Could you check a few things on this model? Use its own coordinates, in mm. A direction names the side the tool comes from. Give positions to 0.01 mm unless a question says otherwise; leave off trailing zeros. Loops run counter-clockwise (first coordinate to the right, second up) from the corner with the lowest first, then second, coordinate; pieces in that order, holes last. Notation, with made-up numbers: M 76,-19.75 L 92,-19.75 A14 ccw 92,-4.75 Z; hole C 62,8.5 d8. An arc over 180 degrees is marked long. Answer in a Markdown table with one row per item. Add a question column.
1. If we section it at A-A on y = 21.5: List the corners of the cut face in (x, z) for me (3 decimals).
2. Thinking about a two-plate mould opening in X: for faces 1 (the flat face through (-4.802, 20, 2)), 2 (the flat face through (25.698, 39, 2)), 3 (the flat face through (32.198, 20, 2)), 4 (the flat face through (13, -6.855, 2)), which applies, released by +X, released by -X, zero draft, split by the parting line, or undercut?
3. I need wall thicknesses on line 1 along Y through (x, z) = (11, 2.7); line 2 along X through (y, z) = (35.5, 0.5); line 3 along Y through (x, z) = (6, 2.4). Which ranges of each line are inside material? Lowest first, please. Write a range as from..to.
4. If we section it at B-B on x = 9.5: List the corners of the cut face in (y, z) for me (3 decimals), then the cut area to 3 significant figures.
5. If we section it at C-C on y = 39: List the corners of the cut face in (x, z) for me (3 decimals).
6. Which directions (+Z, -Z, +X, -X, +Y, -Y) give clear straight access to the entire face, cutting with the end or side of a thin tool? Please do faces 5 (the flat face through (8, 20.82, 2)), 6 (the flat face through (13, 47.32, 2)).
7. If we section it at D-D on x = 23.5: List the corners of the cut face in (y, z) for me (3 decimals).
8. I'm going to push a flat-ended pin straight in: pin 1 Ø1.2 at (x, y) = (-0.8, 11.57) entering from -Z. Where does the tip first touch, or does it pass through?
```python
from build123d import *

# Parameters (mm, degrees)
F0_W     = 37
F0_H     = 54.175
F0_W_2   = 6
F0_H_2   = 3.175
F0_R     = 1
F0_W_3   = 8.325
F0_H_3   = 23.5
F0_W_4   = 10
F0_H_4   = 10
F0_R_2   = 1.2
F1_DEPTH = 3.175


# Not quite as in the source:
# - a length typed as a fraction of an inch, garbled in the dataset ("3 / 203.2 mm" for 3/8 in), is restored
# - a feature names something its author has since deleted; it is built from what else it names


with BuildPart() as f1:
    # F0 (on Top) → F1 (new body)
    with BuildSketch(Plane.XY):
        with Locations((13.6980720539, 20.2328219792)):
            Rectangle(F0_W, F0_H)
        with Locations((5.1980720539, -1.2671780208)):
            Rectangle(F0_W_2, F0_H_2, mode=Mode.SUBTRACT)
        with Locations((-0.8019279461, 11.5703219792)):
            Circle(F0_R, mode=Mode.SUBTRACT)
        with BuildLine():
            ThreePointArc((13.6980720539, 0.2328219792), (14.7587322257, -0.2065178491), (15.1980720539, -1.2671780208))
            ThreePointArc((15.1980720539, -1.2671780208), (12.6374118822, -2.3278381926), (13.6980720539, 0.2328219792))
        make_face(mode=Mode.SUBTRACT)
        with Locations((22.1980720539, -1.2671780208)):
            Rectangle(F0_W_2, F0_H_2, mode=Mode.SUBTRACT)
        Polygon((1.6980720539, 5.3203219792), (1.6980720539, 17.8203219792), (13.6980720539, 17.8203219792), (25.6980720539, 17.8203219792), (25.6980720539, 5.3203219792), align=None, mode=Mode.SUBTRACT)
        with Locations((28.1980720539, 11.5703219792)):
            Circle(F0_R, mode=Mode.SUBTRACT)
        with Locations((8.5355720539, 32.5703219792)):
            Rectangle(F0_W_3, F0_H_3, mode=Mode.SUBTRACT)
        with BuildLine():
            ThreePointArc((-1.8019279461, 42.7328219792), (-0.2144279461, 44.3203219792), (1.3730720539, 42.7328219792))
            Line((1.3730720539, 42.7328219792), (1.3730720539, 29.7328219792))
            ThreePointArc((1.3730720539, 29.7328219792), (-0.2144279461, 28.1453219792), (-1.8019279461, 29.7328219792))
            Line((-1.8019279461, 29.7328219792), (-1.8019279461, 42.7328219792))
        make_face(mode=Mode.SUBTRACT)
        Polygon((15.6980720539, 24.3203219792), (15.6980720539, 34.3203219792), (15.6980720539, 44.3203219792), (25.6980720539, 44.3203219792), (25.6980720539, 34.3203219792), (25.6980720539, 24.3203219792), align=None, mode=Mode.SUBTRACT)
        with Locations((20.6980720539, 29.3203219792)):
            Rectangle(F0_W_4, F0_H_4)
        with Locations((20.6980720539, 29.3203219792)):
            Circle(F0_R_2, mode=Mode.SUBTRACT)
    extrude(amount=F1_DEPTH)


solid = f1.part
```
Results:
| question | item | result |
|---|---|---|
| 1 | outline | M -4.802,0 L 4.373,0 L 4.373,3.175 L -4.802,3.175 Z; M 12.698,0 L 32.198,0 L 32.198,3.175 L 12.698,3.175 Z |
| 2 | face 1 | released by -X |
| 2 | face 2 | undercut |
| 2 | face 3 | released by +X |
| 2 | face 4 | zero draft |
| 3 | line 1 | -6.85..5.32, 17.82..20.82, 44.32..47.32 |
| 3 | line 2 | -4.8..-1.8, 1.37..4.37, 12.7..15.7, 25.7..32.2 |
| 3 | line 3 | -6.85..-2.85, 0.32..5.32, 17.82..20.82, 44.32..47.32 |
| 4 | outline | M -6.855,0 L 5.32,0 L 5.32,3.175 L -6.855,3.175 Z; M 17.82,0 L 20.82,0 L 20.82,3.175 L 17.82,3.175 Z; M 44.32,0 L 47.32,0 L 47.32,3.175 L 44.32,3.175 Z |
| 4 | area | 57.7 mm2 |
| 5 | outline | M -4.802,0 L -1.802,0 L -1.802,3.175 L -4.802,3.175 Z; M 1.373,0 L 4.373,0 L 4.373,3.175 L 1.373,3.175 Z; M 12.698,0 L 15.698,0 L 15.698,3.175 L 12.698,3.175 Z; M 25.698,0 L 32.198,0 L 32.198,3.175 L 25.698,3.175 Z |
| 6 | face 5 | +Z, -Z |
| 6 | face 6 | +Z, -Z, +X, -X, +Y |
| 7 | outline | M -6.855,0 L -2.855,0 L -2.855,3.175 L -6.855,3.175 Z; M 0.32,0 L 5.32,0 L 5.32,3.175 L 0.32,3.175 Z; M 17.82,0 L 34.32,0 L 34.32,3.175 L 17.82,3.175 Z; M 44.32,0 L 47.32,0 L 47.32,3.175 L 44.32,3.175 Z |
| 8 | pin 1 | through |
